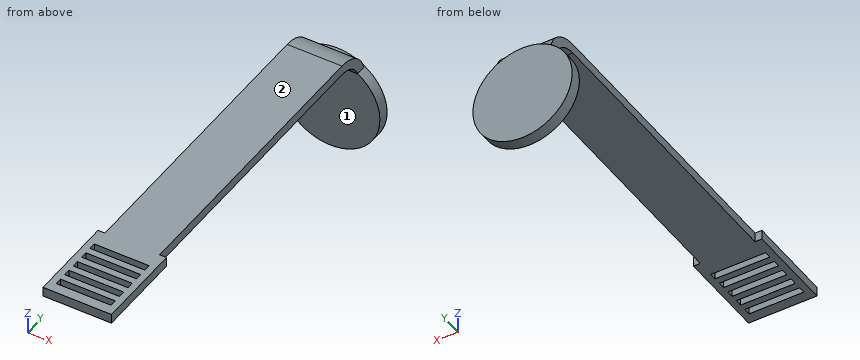
```python
from build123d import *

# Parameters (mm, degrees)
F0_W     = 8
F0_H     = 43
F1_DEPTH = 1.4
F3_DEPTH = 8
F5_R     = 7.25
F6_DEPTH = 1.7
F7_W     = 8
F7_H     = 1
F8_DEPTH = 1.4


with BuildPart() as f1:
    # F0 (on Top) → F1 (new body)
    with BuildSketch(Plane.XY):
        with Locations((0, 28)):
            Rectangle(F0_W, F0_H)
        Polygon((5, -6.5), (5, 6.5), (4, 6.5), (-4, 6.5), (-5, 6.5), (-5, -6.5), align=None)
    extrude(amount=F1_DEPTH)

    # F2 (on face) → F3 (join, through all)
    with BuildSketch(Plane.YZ.offset(4)):
        with BuildLine():
            ThreePointArc((49.5, 0), (52.72945, -1.639777), (53.311111, -5.214674))
            Line((53.311111, -5.214674), (54.9, -4))
            ThreePointArc((54.9, -4), (53.318377, -0.181623), (49.5, 1.4))
            Line((49.5, 1.4), (49.5, 0))
        make_face()
    extrude(amount=-F3_DEPTH)

    # F5 (on face) → F6 (join)
    with BuildSketch(Plane(origin=(0, 54.9, 0), x_dir=(-1, 0, 0), z_dir=(0, 1, 0))):
        with Locations((0, -8.5)):
            Circle(F5_R)
    extrude(amount=-F6_DEPTH)

    # F7 (on face) → F8 (cut, through all)
    with BuildSketch(Plane.XY.offset(1.4)):
        with Locations((0, -4.5)):
            Rectangle(F7_W, F7_H)
        with Locations((0, -2.5)):
            Rectangle(F7_W, F7_H)
        with Locations((0, -0.5)):
            Rectangle(F7_W, F7_H)
        with Locations((0, 1.5)):
            Rectangle(F7_W, F7_H)
        with Locations((0, 3.5)):
            Rectangle(F7_W, F7_H)
    extrude(amount=-F8_DEPTH, mode=Mode.SUBTRACT)


solid = f1.part
```
Can you work these out from the model? Positions are in its coordinate system, mm. Face numbers are marked on the shaded views. A direction names the side the tool comes from. Give positions to 0.01 mm unless a question says otherwise; leave off trailing zeros. Loops run counter-clockwise (first coordinate to the right, second up) from the corner with the lowest first, then second, coordinate; pieces in that order, holes last. Notation, with made-up numbers: M 47,20 L 65,20 A34 cw 65,51 Z; hole C -21,78.5 d2. An arc over 180 degrees is marked long. One line per question, with ' | ' between items. Start each with the question number.
Q1. If we section it at A-A (x = -2.25): State how many separate pieces and enclosed holes the cut face has, plus the area to 3 significant figures.
Q2. If we section it at B-B (z = -8.5): Please give me the cut outline in (x, y), plus the area to 4 significant figures.
Q3. If I drill on line 1 (Y direction, x = -5, z = -7.75); line 2 (Z direction, x = 4.75, y = -2); line 3 (Y direction, x = 0.75, z = -1.25), over which ranges is the centre line in solid material (lowest first)? Write a range as from..to.
Q4. For the marked faces 1 and 2, which set-ups out of +Z, -Z, +X, -X, +Y, -Y let a thin tool reach every point of the face, with its end or its side?
Q5. For pin 1 Ø5 at (y, z) = (29.5, -3.5) entering from +X; pin 2 Ø5 at (x, y) = (-2.5, 43) entering from -Z; pin 3 Ø3 at (y, z) = (32.5, -1) entering from -X; pin 4 Ø0.8 at (y, z) = (3.5, 1) entering from +X, each with a flat end and sliding along its axis, tell me the tip position at first contact or that it passes through.
Q6. If we section it at C-C (y = 22): Please give me the cut outline in (x, z), plus the area to 3 significant figures.
Computed:
1) separate pieces: 6 | enclosed holes: 0 | area: 102 mm²
2) outline: M -7.25,53.2 L 7.25,53.2 L 7.25,54.9 L -7.25,54.9 Z | area: 24.65 mm²
3) line 1: y = 53.2..54.9 | line 2: z = 0..1.4 | line 3: y = 52.4..54.15
4) face 1: -Z, +X, -X, -Y | face 2: +Z, +X, -X, +Y, -Y
5) pin 1: passes through | pin 2: stops at z = 0 | pin 3: stops at x = -4 | pin 4: stops at x = 5
6) outline: M -4,0 L 4,0 L 4,1.4 L -4,1.4 Z | area: 11.2 mm²
